Could you check a few things on this model? Use its own coordinates, in mm. A direction names the side the tool comes from. Give positions to 0.01 mm unless a question says otherwise; leave off trailing zeros. Answer in a Markdown table with one row per item. Add a question column.
```python
from build123d import *

# Parameters (mm, degrees)
SKETCH_2_R          = 2.75
CUT_EXTRUDE_1_DEPTH = 5
SKETCH_3_R          = 6.2
CUT_EXTRUDE_2_DEPTH = 134.492132213


with BuildPart() as part:
    # ｽｹｯﾁ1 → 回転1 (revolve)
    with BuildSketch(Plane.XY, mode=Mode.PRIVATE) as revolve_1_sk:
        with BuildLine():
            Line((-30, 0), (0, 0))
            Line((0, 0), (0, 120))
            Line((0, 120), (-20, 120))
            ThreePointArc((-20, 120), (-40.933866224, 61.327822185), (-30, 0))
        make_face()
    revolve(revolve_1_sk.sketch.rotate(Axis((0, 0, 0), (0, 1, 0)), 270), axis=Axis((0, 0, 0), (0, 1, 0)))

    # ｽｹｯﾁ2 → ｶｯﾄ - 押し出し1 (cut)
    with BuildSketch(Plane(origin=(0, 120, 0), x_dir=(1, 0, 0), z_dir=(0, 1, 0))):
        with Locations(Location((0, 11, 0), (0, 0, 270))):
            Circle(SKETCH_2_R)
        with Locations(Location((9.526279442, -5.5, 0), (0, 0, 270))):
            Circle(SKETCH_2_R)
        with Locations(Location((-9.526279442, -5.5, 0), (0, 0, 270))):
            Circle(SKETCH_2_R)
    cut_extrude_1 = extrude(amount=-CUT_EXTRUDE_1_DEPTH, mode=Mode.SUBTRACT)

    # ﾐﾗｰ1: ｶｯﾄ - 押し出し1 across plane
    add(cut_extrude_1.mirror(Plane.ZX.offset(60)), mode=Mode.SUBTRACT)

    # ｽｹｯﾁ3 → ｶｯﾄ - 押し出し2 (cut, through all)
    with BuildSketch(Plane(origin=(0, 120, 0), x_dir=(1, 0, 0), z_dir=(0, 1, 0))):
        with Locations(Location((0, 0, 0), (0, 0, 270))):
            Circle(SKETCH_3_R)
    extrude(amount=-CUT_EXTRUDE_2_DEPTH, mode=Mode.SUBTRACT)


solid = part.part
```
Item 1: For faces 3 (the face through (0, 115, -11)), 4 (the face through (10, 5, 5)), 5 (the face through (-5, 120, 4)), which set-ups out of +Z, -Z, +X, -X, +Y, -Y let a thin tool reach every point of the face, with its end or its side?
Item 2: If we mould it in two halves opening along X, with no side actions, what happens to faces 1 (the face through (0.83, 117.54, -8.38)), 2 (the face through (0, 0, 7))? For each: +X half, -X half, draft (parallel to the pull), parting line (faces both ways), or undercut.
Item 3: For P1, Ø1.6, axis at x = 8.5, z = 5, coming from the +Y side; P2, Ø5, axis at y = 17, z = 3, coming from the +X side; P3, Ø2, axis at x = -27.5, y = 26.5, coming from the -Z side, each with a flat end and sliding along its axis, tell me the tip position at first contact or that it passes through.
Item 4: I need wall thicknesses on L1, parallel to X at y = 116.75, z = 5.5; L2, parallel to X at y = 118.35, z = 5.5; L3, parallel to X at y = 66, z = -1.5. Which ranges of each line are inside material? Lowest first, please.
Values found:
| question | item | result |
|---|---|---|
| 1 | face 3 | +Y |
| 1 | face 4 | -Y |
| 1 | face 5 | +Z, -Z, +X, -X, +Y |
| 2 | face 1 | undercut |
| 2 | face 2 | draft |
| 3 | P1 | y = 115 |
| 3 | P2 | x = 37.03 |
| 3 | P3 | z = -28.39 |
| 4 | L1 | -21.46 to -12.28, -6.78 to -2.86, 2.86 to 6.78, 12.28 to 21.46 |
| 4 | L2 | -20.39 to -12.28, -6.78 to -2.86, 2.86 to 6.78, 12.28 to 20.39 |
| 4 | L3 | -40.43 to -6.02, 6.02 to 40.43 |
